Part model, mm, in its own coordinate system. Face numbers are marked on the shaded views. A direction names the side the tool comes from. Give positions to 0.01 mm unless a question says otherwise; leave off trailing zeros. Write each loop counter-clockwise with the first axis right and the second up, starting at its lowest first coordinate (ties: lowest second). Pieces come first, ordered by that corner, then holes. Notation, with made-up numbers: M 25.5,66 L 71.5,66 A9 ccw 71.5,80 Z; hole C 24.25,74 d5. An arc over 180 degrees is marked long. Use a Markdown table: item, result.
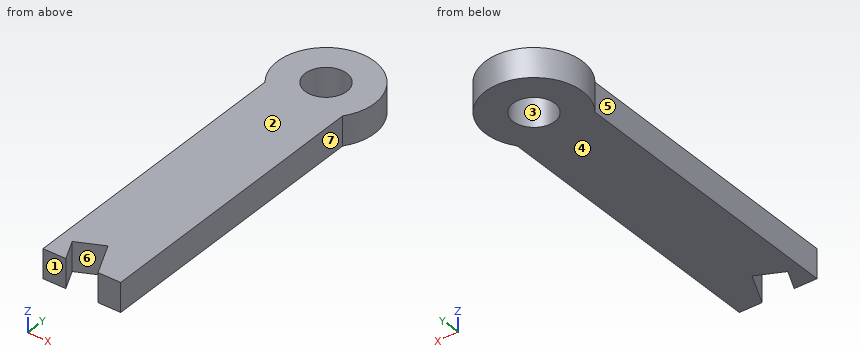
```python
from build123d import *

# Parameters (mm, degrees)
SKETCH1_R           = 2.15
BOSS_EXTRUDE1_DEPTH = 3


with BuildPart() as part:
    # Sketch1 → Boss-Extrude1 (new body)
    with BuildSketch(Plane.XY):
        with BuildLine():
            Line((4, -33), (4, -3))
            ThreePointArc((4, -3), (0, 5), (-4, -3))
            Line((-4, -3), (-4, -33))
            Line((-4, -33), (-1.656379773, -33))
            Line((-1.656379773, -33), (-2.716768264, -30.736026447))
            Line((-2.716768264, -30.736026447), (0, -29.463560258))
            Line((0, -29.463560258), (1.656379773, -33))
            Line((1.656379773, -33), (4, -33))
        make_face()
        Circle(SKETCH1_R, mode=Mode.SUBTRACT)
    extrude(amount=BOSS_EXTRUDE1_DEPTH)


solid = part.part
```
1. Drop flat-ended pins along their axis: P1, Ø1.5, axis at x = 1, z = 2, coming from the +Y side; P2, Ø1.5, axis at y = -13, z = 1.5, coming from the +X side; P3, Ø1.5, axis at y = -6, z = 1.5, coming from the -X side. Give the stop position or say it passes through.
Findings below:
| item | result |
|---|---|
| P1 | y = 4.99 |
| P2 | x = 4 |
| P3 | x = -4 |
2. Two-plate mould, pull along Y, no slides. Class the marked faces 1, 2 and 3: released by +Y, released by -Y, zero draft, split by the parting line, or undercut.
Findings below:
| item | result |
|---|---|
| face 1 | released by -Y |
| face 2 | zero draft |
| face 3 | undercut |
3. Cut at B-B, the plane z = 0.7. Give the cut face in (x, y).
Findings below:
| item | result |
|---|---|
| outline | M -4,-33 L -1.66,-33 L -2.72,-30.74 L 0,-29.46 L 1.66,-33 L 4,-33 L 4,-3 A5 ccw long -4,-3 Z; hole C 0,0 d4.3 |
4. Cut at C-C, the plane x = 0.75. Give the cut face in (y, z), then the cut area to 3 significant figures.
Findings below:
| item | result |
|---|---|
| outline | M -31.06,0 L -2.01,0 L -2.01,3 L -31.06,3 Z; M 2.01,0 L 4.94,0 L 4.94,3 L 2.01,3 Z |
| area | 95.9 mm2 |
5. Tool access for the marked faces 4, 5, 6 and 7: list every direction of +Z, -Z, +X, -X, +Y, -Y with a clear straight run to the whole face (end or side of a thin tool).
Findings below:
| item | result |
|---|---|
| face 4 | -Z, +X, -X, +Y, -Y |
| face 5 | +Z, -Z, -X, -Y |
| face 6 | +Z, -Z |
| face 7 | +Z, -Z, +X, -Y |
6. Cut at D-D, the plane y = -20. Give the cut face in (x, z).
Findings below:
| item | result |
|---|---|
| outline | M -4,0 L 4,0 L 4,3 L -4,3 Z |
7. Cut at A-A, the plane y = 0. Give the cut face in (x, z).
Findings below:
| item | result |
|---|---|
| outline | M -5,0 L -2.15,0 L -2.15,3 L -5,3 Z; M 2.15,0 L 5,0 L 5,3 L 2.15,3 Z |
8. Drill centre lines: L1, parallel to X at y = -6, z = 0.95; L2, parallel to Y at x = -1.5, z = 2.5; L3, parallel to Y at x = 1.75, z = 1.2. Where is each one in solid material? Low to high.
Findings below:
| item | result |
|---|---|
| L1 | -4 to 4 |
| L2 | -30.17 to -1.54, 1.54 to 4.77 |
| L3 | -33 to -1.25, 1.25 to 4.68 |
